Geometry: see drawing. Coordinates: mm, zero at the bounding-box minimum. Coordinates: 2 decimals unless noted, no trailing zeros. Order: outer loops, then holes, each group sorted by start corner. A loop starts at its lowest first (then second) coordinate and runs counter-clockwise, first axis right, second up.
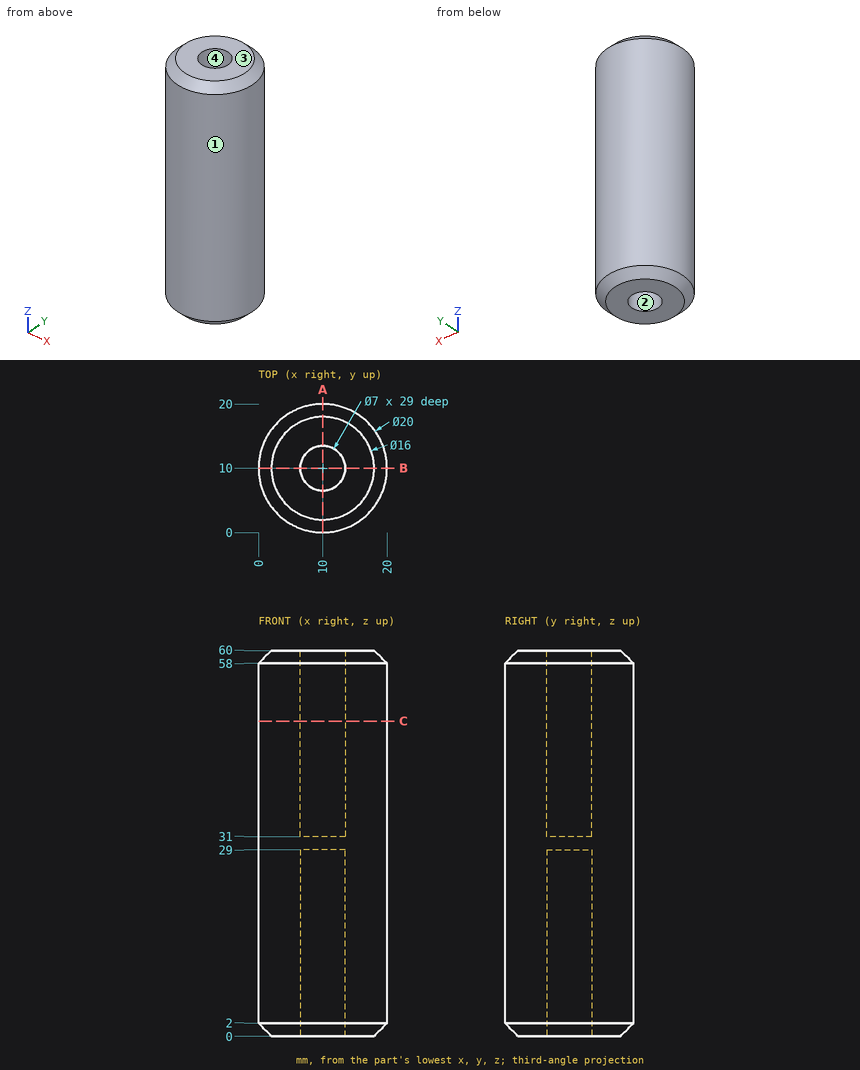
Item 1: Cut plane A-A on x = 10. Return loops of the section in (y, z), then the cut area to 3 significant figures.
Response values:
outline: (0, 2) - (2, 0) - (6.5, 0) - (6.5, 29) - (13.5, 29) - (13.5, 0) - (18, 0) - (20, 2) - (20, 58) - (18, 60) - (13.5, 60) - (13.5, 31) - (6.5, 31) - (6.5, 60) - (2, 60) - (0, 58) - close
area: 786 mm2
Item 2: Draft query along X for the marked faces 1, 2, 3 and 4. Return one class per face: pulls with the +X half, pulls with the -X half, needs draft (parallel to the pull), parting line crosses it, or undercut.
Response values:
face 1: parting line crosses it
face 2: undercut
face 3: needs draft
face 4: undercut
Item 3: Cut plane C-C on z = 49. Return loops of the section in (x, y), then the cut area to 3 significant figures.
Response values:
outline: circle Ø20 at (10, 10); hole circle Ø7 at (10, 10)
area: 276 mm2
Item 4: Pin query (flat end, axial travel): pin 1 Ø6.5 at (x, y) = (10, 10) entering from +Z; pin 2 Ø6 at (y, z) = (4.5, 29.5) entering from -X; pin 3 Ø3 at (x, z) = (5, 20.5) entering from -Y. Return the tip coordinate at first contact, or that it passes through.
Response values:
pin 1: stops at z = 31
pin 2: stops at x = 0.32
pin 3: stops at y = 0.63
Item 5: Ray query, probe 1 along Y at (x, z) = (10, 19); probe 2 along X at (y, z) = (8, 17.5); probe 3 along X at (y, z) = (9.25, 25.5). Return the intervals inside material, ascending.
Response values:
probe 1: y = 0 to 6.5, 13.5 to 20
probe 2: x = 0.2 to 7.13, 12.87 to 19.8
probe 3: x = 0.03 to 6.58, 13.42 to 19.97
